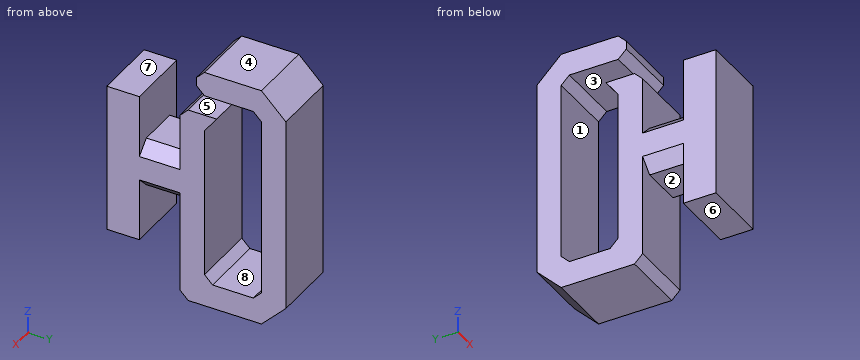
from build123d import *

# Parameters (mm, degrees)
BOSS_EXTRUDE1_DEPTH = 4
CHAMFER1_SIZE       = 0.75
SKETCH2_W           = 1.5
SKETCH2_H           = 1
CUT_EXTRUDE1_DEPTH  = 14.901438774
CHAMFER2_SIZE       = 1.5
CHAMFER3_SIZE       = 0.5


with BuildPart() as part:
    # Sketch1 → Boss-Extrude1 (new body)
    with BuildSketch(Plane(origin=(0, 0, 0), x_dir=(0, 0, -1), z_dir=(1, 0, 0))):
        Polygon((-4.6, 0), (4.6, 0), (4.6, 2), (1.5, 2), (1.5, 4.5), (7.5, 4.5), (7.5, 11), (-7.5, 11), (-7.5, 4.5), (-6, 4.5), (-6, 6), (-6, 9.5), (6, 9.5), (6, 6), (-3.75, 6), (-4.75, 6.75), (-4.75, 6), (-4.75, 4.5), (-1.5, 4.5), (-1.5, 2), (-4.6, 2), align=None)
    extrude(amount=BOSS_EXTRUDE1_DEPTH)

    # Chamfer1
    chamfer1_edges = [part.edges().sort_by_distance(p)[0] for p in [
        (0, 3.25, 1.5),
        (0, 3.25, -1.5),
        (4, 3.25, 1.5),
        (4, 3.25, -1.5),
    ]]
    chamfer(chamfer1_edges, length=CHAMFER1_SIZE)

    # Sketch2 → Cut-Extrude1 (cut, through all)
    with BuildSketch(Plane.ZY):
        with Locations((6.75, 5)):
            Rectangle(SKETCH2_W, SKETCH2_H)
    extrude(amount=-CUT_EXTRUDE1_DEPTH, mode=Mode.SUBTRACT)

    # Chamfer2
    chamfer2_edges = [part.edges().sort_by_distance(p)[0] for p in [
        (2, 11, 7.5),
        (2, 11, -7.5),
    ]]
    chamfer(chamfer2_edges, length=CHAMFER2_SIZE)

    # Chamfer3
    chamfer3_edges = [part.edges().sort_by_distance(p)[0] for p in [
        (2, 5.5, 6),
        (2, 5.5, 7.5),
        (2, 4.5, 4.75),
        (2, 6, -6),
        (2, 9.5, -6),
        (2, 9.5, 6),
        (2, 4.5, -7.5),
    ]]
    chamfer(chamfer3_edges, length=CHAMFER3_SIZE)


solid = part.part
Part model, mm, in its own coordinate system. Face numbers are marked on the shaded views. A direction names the side the tool comes from. Round coordinates to 2 decimals unless told otherwise and drop trailing zeros. Write each loop counter-clockwise with the first axis right and the second up, starting at its lowest first coordinate (ties: lowest second). Pieces come first, ordered by that corner, then holes. Notation, with made-up numbers: M 61.25,-38 L 83.25,-38 A16 ccw 83.25,-10 Z; hole C 25.5,73.25 d8. An arc over 180 degrees is marked long. Return JSON: item names as keys, results as strings. Group by question number.
(1) Saw through at A-A on y = 7.25. Write the cut outline in (x, z), then the cut area to 3 significant figures.
(2) Drill centre lines: probe 1 along Y at (x, z) = (1.25, 2.75); probe 2 along Z at (x, y) = (1.75, 8.5); probe 3 along Z at (x, y) = (1.8, 3.75). Where is each one in solid material? Low to high.
(3) Two-plate mould, pull along Z, no slides. Class the marked faces 1, 2, 3 and 4: +Z half, -Z half, draft (parallel to the pull), parting line (faces both ways), or undercut.
(4) Which spindle directions (+Z, -Z, +X, -X, +Y, -Y) get a long thin tool onto all of the face, cutting with end or side? Do the marked faces 5, 6, 7 and 8. Say none if no direction does.
(5) Pin check, flat tips, straight feed: pin 1 Ø2 at (x, y) = (1.5, 1) entering from +Z; pin 2 Ø1.5 at (x, z) = (2, -5.5) entering from -Y; pin 3 Ø0.6 at (x, z) = (1.5, 6.5) entering from -Y. Stop position of each tip, or through.
(6) Saw through at D-D on z = -1.25. Write the cut outline in (x, y), then the cut area to 3 significant figures.
(7) Saw through at C-C on x = 1.6. Write the cut outline in (y, z), then the cut area to 3 significant figures.
(8) Saw through at B-B on z = -2.75. Write the cut outline in (x, y).
Returned:
{
 "1": {"outline": "M 0,-7.5 L 4,-7.5 L 4,-6 L 0,-6 Z; M 0,6 L 4,6 L 4,7.5 L 0,7.5 Z", "area": "12.0 mm²"},
 "2": {"probe 1": "0 to 2, 4.5 to 6, 9.5 to 11", "probe 2": "-7.5 to -6, 6 to 7.5", "probe 3": "-1.5 to 1.5"},
 "3": {"face 1": "undercut", "face 2": "-Z half", "face 3": "undercut", "face 4": "+Z half"},
 "4": {"face 5": "+X, -X, -Y", "face 6": "-Z, +X, -X, -Y", "face 7": "+Z, +X, -X, -Y", "face 8": "+X, -X"},
 "5": {"pin 1": "z = 4.6", "pin 2": "y = 4.5", "pin 3": "y = 5.5"},
 "6": {"outline": "M 0,0 L 4,0 L 4,2 L 3.5,2 L 3.5,4.5 L 4,4.5 L 4,6 L 0,6 L 0,4.5 L 0.5,4.5 L 0.5,2 L 0,2 Z; M 0,9.5 L 4,9.5 L 4,11 L 0,11 Z", "area": "27.5 mm²"},
 "7": {"outline": "M 0,-4.6 L 2,-4.6 L 2,-1.5 L 4.5,-1.5 L 4.5,-7 L 5,-7.5 L 9.5,-7.5 L 11,-6 L 11,6 L 9.5,7.5 L 6,7.5 L 5.5,7 L 5.5,6.5 L 6,6 L 9,6 L 9.5,5.5 L 9.5,-5.5 L 9,-6 L 6.5,-6 L 6,-5.5 L 6,3.75 L 6.75,4.75 L 5,4.75 L 4.5,4.25 L 4.5,1.5 L 2,1.5 L 2,4.6 L 0,4.6 Z", "area": "76.0 mm²"},
 "8": {"outline": "M 0,0 L 4,0 L 4,2 L 0,2 Z; M 0,4.5 L 4,4.5 L 4,6 L 0,6 Z; M 0,9.5 L 4,9.5 L 4,11 L 0,11 Z"}
}
